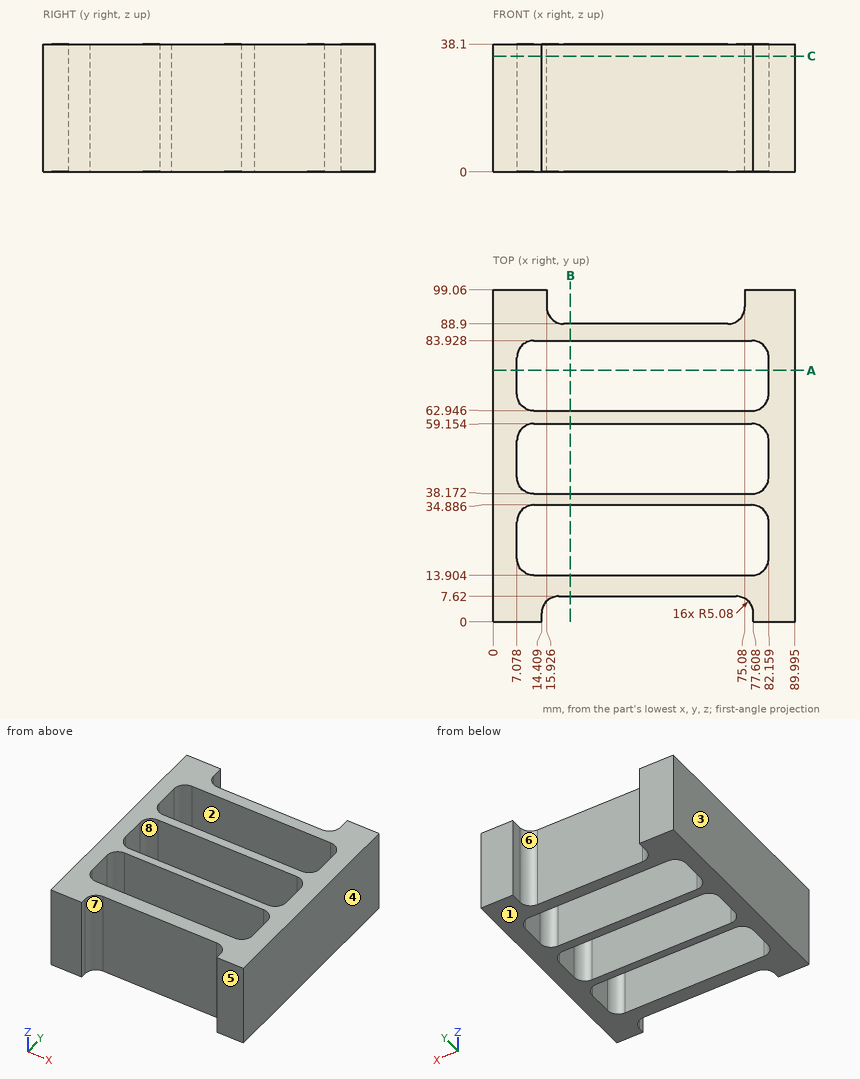
Job drawing, mm, ordinate dimensions from the low corner. One solid piece. A direction names the side the tool comes from. Give positions to 0.01 mm unless a question says otherwise; leave off trailing zeros. Write each loop counter-clockwise with the first axis right and the second up, starting at its lowest first coordinate (ties: lowest second). Pieces come first, ordered by that corner, then holes. Notation, with made-up numbers: (1.25, -11.75) - (11.25, -11.75) arc R28 cw to (11.25, 20.25) - close; hole circle Ø6 at (-5, -37.5). An arc over 180 degrees is marked (long way). Use one line per item in the form item = value. Start each with the question number.
1. 3-axis set-ups, long thin cutter, end or side, ignore diameter. For the marked faces 4, 5, 6, 7 and 8: which of +Z, -Z, +X, -X, +Y, -Y reach the whole face in a straight line?
2. Band-saw the part on C-C on z = 34.5. Count the separate pieces of the cut face and the enclosed holes in it.
3. Probe line 1 (Y direction, x = 46.5, z = 8) (1 decimal); line 2 (Y direction, x = 12.5, z = 36) (1 decimal); line 3 (X direction, y = 54, z = 24.5) (1 decimal). List the from-to ranges inside material, lowest first. Write a range as [from, to].
4. Two-plate mould, pull along X, no slides. Class the marked faces 1, 2 and 3: released by +X, released by -X, zero draft, split by the parting line, or undercut.
5. Drop flat-ended pins along their axis: pin 1 Ø11.5 at (x, z) = (37, 19.5) entering from -Y; pin 2 Ø5 at (x, z) = (46.5, 6.5) entering from +Y. Give the stop position or say it passes through.
6. Band-saw the part on A-A on y = 75. Write the cut outline in (x, z) (1 decimal).
7. Band-saw the part on B-B on x = 23. Write the cut outline in (y, z) (1 decimal).
Conclusion:
q1.face_4 = +Z, -Z, +X, +Y, -Y
q1.face_5 = +Z, -Z, +X, -X, -Y
q1.face_6 = +Z, -Z, +Y
q1.face_7 = +Z, -Z, -Y
q1.face_8 = +Z, -Z
q2.separate_pieces = 1
q2.enclosed_holes = 3
q3.line_1 = [7.6, 13.9], [34.9, 38.2], [59.2, 62.9], [83.9, 88.9]
q3.line_2 = [0, 13.9], [34.9, 38.2], [59.2, 62.9], [83.9, 99.1]
q3.line_3 = [0, 7.1], [82.2, 90]
q4.face_1 = zero draft
q4.face_2 = undercut
q4.face_3 = released by -X
q5.pin_1 = 7.62
q5.pin_2 = 88.9
q6.outline = (0, 0) - (7.1, 0) - (7.1, 38.1) - (0, 38.1) - close; (82.2, 0) - (90, 0) - (90, 38.1) - (82.2, 38.1) - close
q7.outline = (7.6, 0) - (13.9, 0) - (13.9, 38.1) - (7.6, 38.1) - close; (34.9, 0) - (38.2, 0) - (38.2, 38.1) - (34.9, 38.1) - close; (59.2, 0) - (62.9, 0) - (62.9, 38.1) - (59.2, 38.1) - close; (83.9, 0) - (88.9, 0) - (88.9, 38.1) - (83.9, 38.1) - close
